```python
from build123d import *

# Parameters (mm, degrees)
F0_W      = 18
F0_H      = 18
F1_DEPTH  = 7.874
F4_DEPTH  = 25
F5_DEPTH  = 25
F6_T      = -1.6
F7_R      = 2.77
F8_DEPTH  = 7
F10_DEPTH = 3
F12_DEPTH = 0.2
F13_DEPTH = 1
F14_DEPTH = 1


with BuildPart() as f1:
    # F0 (on Top) → F1 (new body)
    with BuildSketch(Plane.XY):
        Rectangle(F0_W, F0_H)
    extrude(amount=F1_DEPTH)

    # F3 (on face) → F4 (cut)
    with BuildSketch(Plane(origin=(-9, 0, 0), x_dir=(0, -1, 0), z_dir=(-1, 0, 0))):
        with BuildLine():
            Line((-6, 7.874), (-9, 7.874))
            Line((-9, 7.874), (-7.232233047, 6.106233047))
            ThreePointArc((-7.232233047, 6.106233047), (-6.6524748606, 7.0154603305), (-6, 7.874))
        make_face()
        with BuildLine():
            Line((-7.232233047, 6.106233047), (-9, 7.874))
            Line((-9, 7.874), (-9, 0))
            ThreePointArc((-9, 0), (-8.491581374, 3.1618143655), (-7.232233047, 6.106233047))
        make_face()
        with BuildLine():
            Line((0, 7.874), (-6, 7.874))
            ThreePointArc((-6, 7.874), (-3.0203476621, 7.3495914676), (0, 7.174))
            Line((0, 7.174), (0, 7.874))
        make_face()
        with BuildLine():
            Line((0, 7.874), (0, 7.174))
            ThreePointArc((0, 7.174), (3.0203476621, 7.3495914676), (6, 7.874))
            Line((6, 7.874), (0, 7.874))
        make_face()
        with BuildLine():
            Line((9, 7.874), (6, 7.874))
            ThreePointArc((6, 7.874), (6.6524748606, 7.0154603305), (7.232233047, 6.106233047))
            Line((7.232233047, 6.106233047), (9, 7.874))
        make_face()
        with BuildLine():
            ThreePointArc((7.232233047, 6.106233047), (8.491581374, 3.1618143655), (9, 0))
            Line((9, 0), (9, 7.874))
            Line((9, 7.874), (7.232233047, 6.106233047))
        make_face()
    extrude(amount=-F4_DEPTH, mode=Mode.SUBTRACT)

    # F2 (on face) → F5 (cut)
    with BuildSketch(Plane.XZ.offset(9)):
        with BuildLine():
            Line((-7.232233047, 6.106233047), (-9, 7.874))
            Line((-9, 7.874), (-9, 0))
            ThreePointArc((-9, 0), (-8.491581374, 3.1618143655), (-7.232233047, 6.106233047))
        make_face()
        with BuildLine():
            Line((-6, 7.874), (-9, 7.874))
            Line((-9, 7.874), (-7.232233047, 6.106233047))
            ThreePointArc((-7.232233047, 6.106233047), (-6.6524748606, 7.0154603305), (-6, 7.874))
        make_face()
        with BuildLine():
            Line((6, 7.874), (0, 7.874))
            Line((0, 7.874), (0, 7.174))
            ThreePointArc((0, 7.174), (3.0203476621, 7.3495914676), (6, 7.874))
        make_face()
        with BuildLine():
            Line((0, 7.874), (-6, 7.874))
            ThreePointArc((-6, 7.874), (-3.0203476621, 7.3495914676), (0, 7.174))
            Line((0, 7.174), (0, 7.874))
        make_face()
        with BuildLine():
            Line((9, 7.874), (6, 7.874))
            ThreePointArc((6, 7.874), (6.6524748606, 7.0154603305), (7.232233047, 6.106233047))
            Line((7.232233047, 6.106233047), (9, 7.874))
        make_face()
        with BuildLine():
            ThreePointArc((7.232233047, 6.106233047), (8.491581374, 3.1618143655), (9, 0))
            Line((9, 0), (9, 7.874))
            Line((9, 7.874), (7.232233047, 6.106233047))
        make_face()
    extrude(amount=-F5_DEPTH, mode=Mode.SUBTRACT)

    # F6
    f6_openings = [f1.faces().sort_by_distance(p)[0] for p in [
        (0, 0, 0),
    ]]
    offset(amount=F6_T, openings=f6_openings)

    # F7 (on face) → F8 (join)
    with BuildSketch(Plane(origin=(0, 0, 0), x_dir=(1, 0, 0), z_dir=(0, 0, -1))):
        Circle(F7_R)
        Polygon((0.7, 2.1), (0.7, 0.7), (2.1, 0.7), (2.1, 0), (2.1, -0.7), (0.7, -0.7), (0.7, -2.1), (0, -2.1), (-0.7, -2.1), (-0.7, -0.7), (-2.1, -0.7), (-2.1, 0), (-2.1, 0.7), (-0.7, 0.7), (-0.7, 2.1), (0, 2.1), align=None, mode=Mode.SUBTRACT)
    extrude(amount=-F8_DEPTH)

    # F9 (on face) → F10 (cut)
    with BuildSketch(Plane(origin=(0, 0, 0), x_dir=(1, 0, 0), z_dir=(0, 0, -1))):
        with BuildLine():
            Line((-2.1, -0.7), (-2.1, 0.7))
            Line((-2.1, 0.7), (-2.680093282, 0.7))
            ThreePointArc((-2.680093282, 0.7), (-2.77, 0), (-2.680093282, -0.7))
            Line((-2.680093282, -0.7), (-2.1, -0.7))
        make_face()
        with BuildLine():
            ThreePointArc((2.77, 0), (2.7474313814, 0.3528750551), (2.680093282, 0.7))
            Line((2.680093282, 0.7), (2.1, 0.7))
            Line((2.1, 0.7), (2.1, -0.7))
            Line((2.1, -0.7), (2.680093282, -0.7))
            ThreePointArc((2.680093282, -0.7), (2.7474313814, -0.3528750551), (2.77, 0))
        make_face()
    extrude(amount=-F10_DEPTH, mode=Mode.SUBTRACT)

    # F11 (on face) → F12 (join)
    with BuildSketch(Plane(origin=(0, 0, 0), x_dir=(1, 0, 0), z_dir=(0, 0, -1))):
        with BuildLine():
            ThreePointArc((-2.680093282, 0.7), (0, 2.77), (2.680093282, 0.7))
            Line((2.680093282, 0.7), (2.680093282, 6.7))
            Line((2.680093282, 6.7), (-2.680093282, 6.7))
            Line((-2.680093282, 6.7), (-2.680093282, 0.7))
        make_face()
        Polygon((-0.700093282, -0.7), (-2.680093282, -0.7), (-2.680093282, -6.7), (2.679906718, -6.7), (2.679906718, -0.7), (0.699906718, -0.7), (0.699906718, -2.1), (-0.700093282, -2.1), align=None)
    extrude(amount=-F12_DEPTH)

    # F13 (add): a face of the model
    f13_faces = [f1.faces().sort_by_distance(p)[0] for p in [
        (0, -6.7, 0.1),
    ]]
    extrude(f13_faces, amount=F13_DEPTH)

    # F14 (add): a face of the model
    f14_faces = [f1.faces().sort_by_distance(p)[0] for p in [
        (-9.3282e-05, 6.7, 0.1),
    ]]
    extrude(f14_faces, amount=F14_DEPTH)


solid = f1.part
```
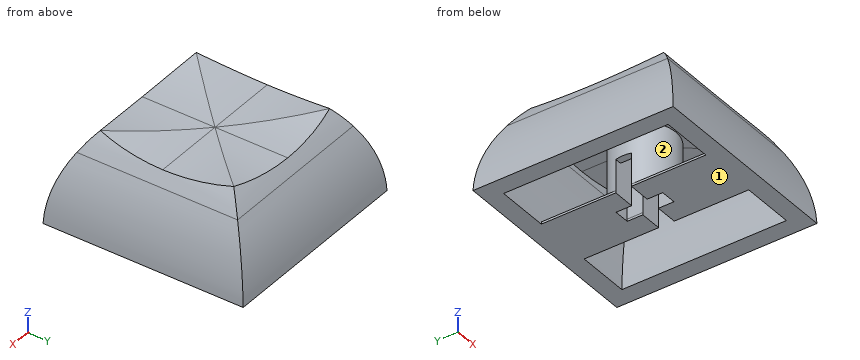
Could you check a few things on this model? Use its own coordinates, in mm. Face numbers are marked on the shaded views. Round coordinates to 2 decimals unless told otherwise and drop trailing zeros. Loops run counter-clockwise (first coordinate to the right, second up) from the corner with the lowest first, then second, coordinate; pieces in that order, holes last. Notation, with made-up numbers: (-8.75, 49.25) -> (22.25, 49.25) arc R19 ccw to (22.25, 71.25) -> close; hole circle Ø4 at (6, -31.75). An arc over 180 degrees is marked (long way). One line per question, with ' | ' between items.
(1) If we section it at C-C on x = 4.25: List the corners of the cut face in (y, z) for me.
Model answer:
outline: (-9, 0) -> (-7.4, 0) arc R11.52 cw to (-5.47, 5.9) -> (-4.25, 5.9) arc R27.66 ccw to (4.25, 5.9) -> (5.47, 5.9) arc R11.52 cw to (7.4, 0) -> (9, 0) arc R13.12 ccw to (6.28, 7.52) -> (4.25, 7.52) arc R26.06 cw to (-4.25, 7.52) -> (-6.28, 7.52) arc R13.12 ccw to start
(2) If I drill on probe 1 along Y at (x, z) = (1.25, 0.75); probe 2 along Y at (x, z) = (-2.5, 1.5); probe 3 along X at (y, z) = (-0.5, 5.5), over which ranges is the centre line in solid material (lowest first)?
Model answer:
probe 1: y = -8.95 to -7.34, -2.47 to -0.7, 0.7 to 2.47, 7.34 to 8.95 | probe 2: y = -8.86 to -7.24, -1.19 to -0.7, 0.7 to 1.19, 7.24 to 8.86 | probe 3: x = -7.56 to -5.73, -2.72 to -2.1, 2.1 to 2.72, 5.73 to 7.56
(3) If we section it at A-A on z = 4: List the corners of the cut face in (x, y) for me, and give its area (3 significant figures).
Model answer:
outline: (-8.22, -8.22) -> (8.22, -8.22) -> (8.22, 8.22) -> (-8.22, 8.22) -> close; circle Ø5.54 at (0, 0); hole (-6.5, -6.5) -> (6.5, -6.5) -> (6.5, 6.5) -> (-6.5, 6.5) -> close; hole (-2.1, -0.7) -> (-0.7, -0.7) -> (-0.7, -2.1) -> (0.7, -2.1) -> (0.7, -0.7) -> (2.1, -0.7) -> (2.1, 0.7) -> (0.7, 0.7) -> (0.7, 2.1) -> (-0.7, 2.1) -> (-0.7, 0.7) -> (-2.1, 0.7) -> close | area: 115 mm^2
(4) If we section it at D-D on y = 2.5: List the corners of the cut face in (x, z) for me.
Model answer:
outline: (-9, 0) -> (-7.4, 0) arc R11.52 cw to (-5.61, 5.69) -> (-2.5, 5.69) arc R27.66 ccw to (-1.19, 5.6) -> (-1.19, 0.2) -> (-2.68, 0.2) -> (-2.68, 0) -> (2.68, 0) -> (2.68, 0.2) -> (1.19, 0.2) -> (1.19, 5.6) arc R27.66 ccw to (2.5, 5.69) -> (5.61, 5.69) arc R11.52 cw to (7.4, 0) -> (9, 0) arc R13.12 ccw to (6.45, 7.29) -> (2.5, 7.29) arc R26.06 cw to (-2.5, 7.29) -> (-6.45, 7.29) arc R13.12 ccw to start
(5) For pin 1 Ø10 at (x, y) = (-7, -3) entering from +Z; pin 2 Ø1.6 at (x, z) = (-2, 3.5) entering from -Y; pin 3 Ø0.7 at (x, y) = (-2.5, 0) entering from -Z; pin 4 Ø1.5 at (x, z) = (-5.5, 6.5) entering from +Y, each with a flat end and sliding along its axis, tell me the tip position at first contact or that it passes through.
Model answer:
pin 1: stops at z = 7.87 | pin 2: stops at y = -8.62 | pin 3: stops at z = 3 | pin 4: stops at y = 7.43
(6) If we section it at B-B on z = 1.5: List the corners of the cut face in (x, y) for me.
Model answer:
outline: (-8.86, -8.86) -> (8.86, -8.86) -> (8.86, 8.86) -> (-8.86, 8.86) -> close; (-2.68, -0.7) arc R2.77 ccw to (2.68, -0.7) -> (0.7, -0.7) -> (0.7, -2.1) -> (-0.7, -2.1) -> (-0.7, -0.7) -> close; (-2.68, 0.7) -> (-0.7, 0.7) -> (-0.7, 2.1) -> (0.7, 2.1) -> (0.7, 0.7) -> (2.68, 0.7) arc R2.77 ccw to start; hole (-7.24, -7.24) -> (7.24, -7.24) -> (7.24, 7.24) -> (-7.24, 7.24) -> close
(7) Thinking about a two-plate mould opening in Z: for the marked faces 1 and 2, which applies, released by +Z, released by -Z, zero draft, split by the parting line, or undercut?
Model answer:
face 1: released by -Z | face 2: undercut
